Geometry check sheet. Reference: the model listing, model coordinates, mm. Face numbers are marked on the shaded views. A direction names the side the tool comes from. Round coordinates to 2 decimals unless told otherwise and drop trailing zeros. Write each loop counter-clockwise with the first axis right and the second up, starting at its lowest first coordinate (ties: lowest second). Pieces come first, ordered by that corner, then holes. Notation, with made-up numbers: M 17.25,16.25 L 71.25,16.25 A23 cw 71.25,40.25 Z; hole C -39,-10 d6. An arc over 180 degrees is marked long. Put each result on its own line as item: value. Start each with the question number.
(1) Gauge pin test, flat ends, axial feed: pin 1 (16.5 mm diameter, centred on x = 7.5, y = 26, fed in from +Z) (3 decimals); pin 2 (10 mm diameter, centred on x = 86, z = 58, fed in from +Y); pin 3 (8 mm diameter, centred on x = 56.5, z = 59, fed in from +Y). Record the tip position at first contact, or that the pin passes through.
(2) Section check C-C on y = -55. Record the cut outline in (x, z) (3 decimals), then the cut area to 3 significant figures.
(3) Section check A-A on y = -23. Record the cut outline in (x, z) (3 decimals).
(4) Material ranges on probe 1 along Y at (x, z) = (38.5, 22); probe 2 along Z at (x, y) = (63, -23) (3 decimals); probe 3 along X at (y, z) = (14.5, 7.5) (3 decimals), recorded low to high.
(5) Tool access check on the marked faces 1, 2 and 3. Record the directions out of +Z, -Z, +X, -X, +Y, -Y that give a thin tool (end or side, any length) a straight path to the whole face; none if there is none.
(6) Section check B-B on x = 95.5. Record the cut outline in (y, z) (3 decimals).
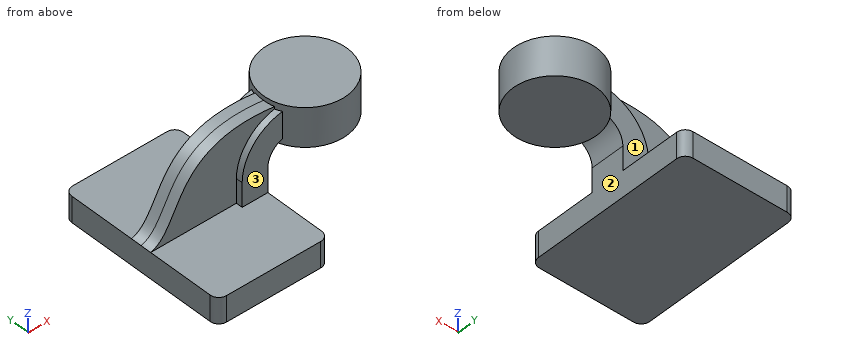
from build123d import *

# Parameters (mm, degrees)
F1_DEPTH = 63.5
F2_DEPTH = 12.7
F3_DEPTH = 7.9375
F0_W     = 30.857466
F0_H     = 28.575
F5_R     = 6.35


with BuildPart() as f1:
    # F0 (on Front) → F1 (new body, symmetric)
    with BuildSketch(Plane.XZ):
        Polygon((41.275, -9.525), (41.275, 9.525), (22.225, 9.525), (-41.275, 9.525), (-41.275, -9.525), align=None)
    extrude(amount=F1_DEPTH, both=True)

    # F0 (on Front) → F2 (join, symmetric)
    with BuildSketch(Plane.XZ):
        Polygon((60.325, 62.183225), (60.325, 43.133225), (60.325, 38.1), (80.267534, 38.1), (80.267534, 66.675), (60.325, 66.675), align=None)
        with BuildLine():
            Line((22.225, 9.525), (41.275, 9.525))
            Line((41.275, 9.525), (41.275, 27.258225))
            ThreePointArc((41.275, 27.258225), (45.92468, 38.483545), (57.15, 43.133225))
            Line((57.15, 43.133225), (60.325, 43.133225))
            Line((60.325, 43.133225), (60.325, 62.183225))
            Line((60.325, 62.183225), (57.15, 62.183225))
            ThreePointArc((57.15, 62.183225), (32.454296, 51.953929), (22.225, 27.258225))
            Line((22.225, 27.258225), (22.225, 9.525))
        make_face()
    extrude(amount=F2_DEPTH, both=True)

    # F0 (on Front) → F3 (join, symmetric)
    with BuildSketch(Plane.XZ):
        with BuildLine():
            Line((-41.275, 9.525), (22.225, 9.525))
            Line((22.225, 9.525), (22.225, 27.258225))
            ThreePointArc((22.225, 27.258225), (32.454296, 51.953929), (57.15, 62.183225))
            add(Edge.make_bspline(
                [(-41.275, 9.525), (-16.467026, 16.406592), (-27.628707, 77.485785), (57.15, 62.183225)],
                knots=[0, 0, 0, 0, 111.626024, 111.626024, 111.626024, 111.626024], degree=3))
        make_face()
    extrude(amount=F3_DEPTH, both=True)

    # F0 (on Front) → F4 (revolve)
    with BuildSketch(Plane.XZ):
        with Locations((95.696267, 52.3875)):
            Rectangle(F0_W, F0_H)
    revolve(axis=Axis((80.267534, 0, 52.3875), (0, 0, 1)))

    # F5
    f5_edges = [f1.edges().sort_by_distance(p)[0] for p in [
        (-41.275, -63.5, 0),
        (41.275, -63.5, 0),
        (41.275, 63.5, 0),
        (-41.275, 63.5, 0),
    ]]
    fillet(f5_edges, radius=F5_R)


solid = f1.part
Answers follow:
1. pin 1: stops at z = 9.525
1. pin 2: stops at y = 30.85
1. pin 3: stops at y = 23.69
2. outline: M -41.275,-9.525 L 41.275,-9.525 L 41.275,9.525 L -41.275,9.525 Z
2. area: 1,570 mm^2
3. outline: M -41.275,-9.525 L 41.275,-9.525 L 41.275,9.525 L -41.275,9.525 Z; M 59.696,38.1 L 100.839,38.1 L 100.839,66.675 L 59.696,66.675 Z
4. probe 1: y = -12.7 to 12.7
4. probe 2: z = 38.1 to 66.675
4. probe 3: x = -41.275 to 41.275
5. face 1: +Z, -X, +Y
5. face 2: -Z, +X, +Y, -Y
5. face 3: +Z, -X, -Y
6. outline: M -26.836,38.1 L 26.836,38.1 L 26.836,66.675 L -26.836,66.675 Z
